Can you work these out from the drawing? Everything is in mm from the part's minimum corner. A direction names the side the tool comes from. Round coordinates to 2 decimals unless told otherwise and drop trailing zeros. Loops run counter-clockwise (first coordinate to the right, second up) from the corner with the lowest first, then second, coordinate; pieces in that order, holes last. Notation, with made-up numbers: (56.5, 39) -> (87.5, 39) arc R29 cw to (87.5, 74) -> close; hole circle Ø11 at (-15.75, 72). An arc over 180 degrees is marked (long way). One line per item, written item: value.
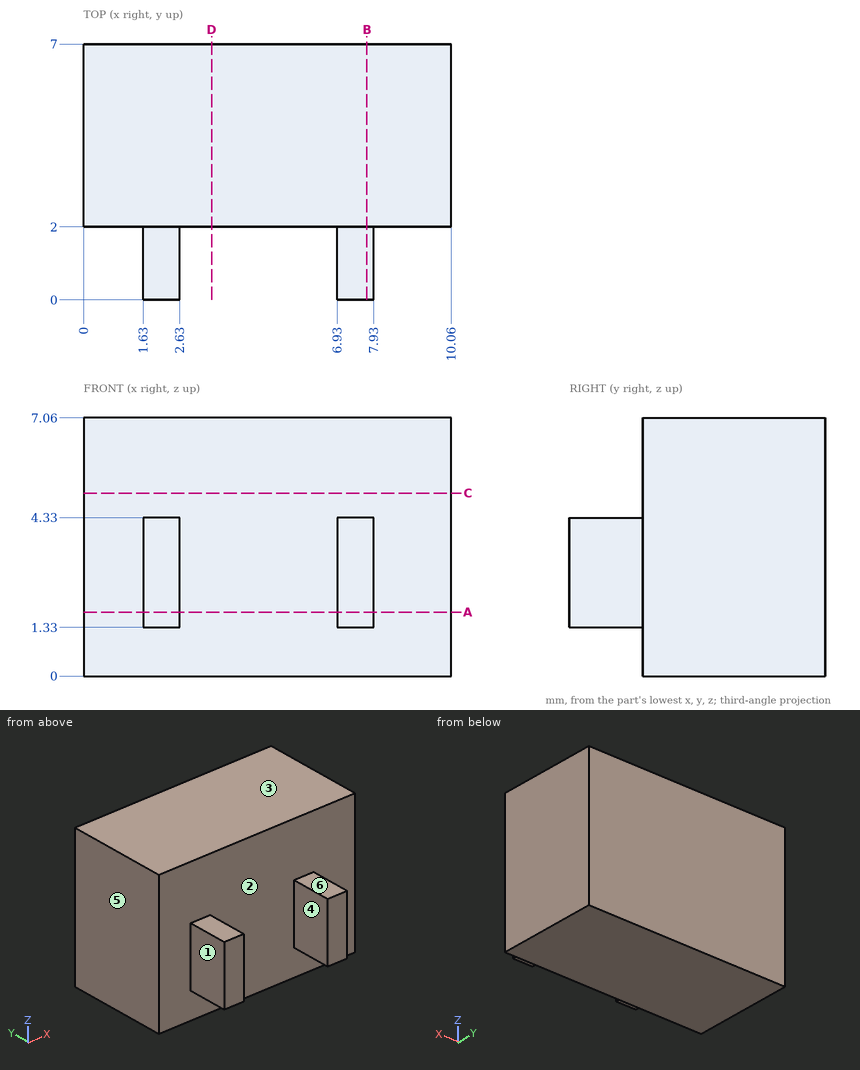
Item 1: For the marked faces 5 and 6, which set-ups out of +Z, -Z, +X, -X, +Y, -Y let a thin tool reach every point of the face, with its end or its side?
Output:
face 5: +Z, -Z, -X, +Y, -Y
face 6: +Z, +X, -X, -Y
Item 2: If we section it at A-A on z = 1.75: List the corners of the cut face in (x, y) for me, plus the area to 3 significant figures.
Output:
outline: (0, 2) -> (1.63, 2) -> (1.63, 0) -> (2.63, 0) -> (2.63, 2) -> (6.93, 2) -> (6.93, 0) -> (7.93, 0) -> (7.93, 2) -> (10.06, 2) -> (10.06, 7) -> (0, 7) -> close
area: 54.3 mm²
Item 3: If we section it at D-D on x = 3.5: List the corners of the cut face in (y, z) for me, plus the area to 3 significant figures.
Output:
outline: (2, 0) -> (7, 0) -> (7, 7.06) -> (2, 7.06) -> close
area: 35.3 mm²
Item 4: If we section it at B-B on x = 7.75: List the corners of the cut face in (y, z) for me.
Output:
outline: (0, 1.33) -> (2, 1.33) -> (2, 0) -> (7, 0) -> (7, 7.06) -> (2, 7.06) -> (2, 4.33) -> (0, 4.33) -> close
Item 5: Will these pins go through, and if not, where does the flat tip stop? pin 1 Ø3 at (x, z) = (3.5, 2) entering from -Y; pin 2 Ø1 at (y, z) = (1, 2) entering from +X; pin 3 Ø2 at (y, z) = (0.5, 3.5) entering from -X; pin 4 Ø1.1 at (x, y) = (2, 0.5) entering from -Z.
Output:
pin 1: stops at y = 0
pin 2: stops at x = 7.93
pin 3: stops at x = 1.63
pin 4: stops at z = 1.33
Item 6: If we mould it in two halves opening along X, with no side actions, what happens to the marked faces 1, 2, 3 and 4? For each: released by +X, released by -X, zero draft, split by the parting line, or undercut.
Output:
face 1: released by -X
face 2: undercut
face 3: zero draft
face 4: undercut
Item 7: I need wall thicknesses on line 1 (X direction, y = 1.25, z = 1.5); line 2 (Y direction, x = 1.5, z = 1.5). Which ranges of each line are inside material? Lowest first, please. Write a range as from..to.
Output:
line 1: x = 1.63..2.63, 6.93..7.93
line 2: y = 2..7
Item 8: If we section it at C-C on z = 5: List the corners of the cut face in (x, y) for me.
Output:
outline: (0, 2) -> (10.06, 2) -> (10.06, 7) -> (0, 7) -> close
